Can you work these out from the drawing? Everything is in mm from the part's minimum corner. Coordinates: 2 decimals unless noted, no trailing zeros. Order: outer loops, then holes, each group sorted by start corner. A loop starts at its lowest first (then second) coordinate and runs counter-clockwise, first axis right, second up. Notation, with made-up numbers: M 28,71 L 67,71 A20 cw 67,95 Z; hole C 9.25,9.25 d11. An arc over 180 degrees is marked long. Answer as a JSON object with one key per item and string values.
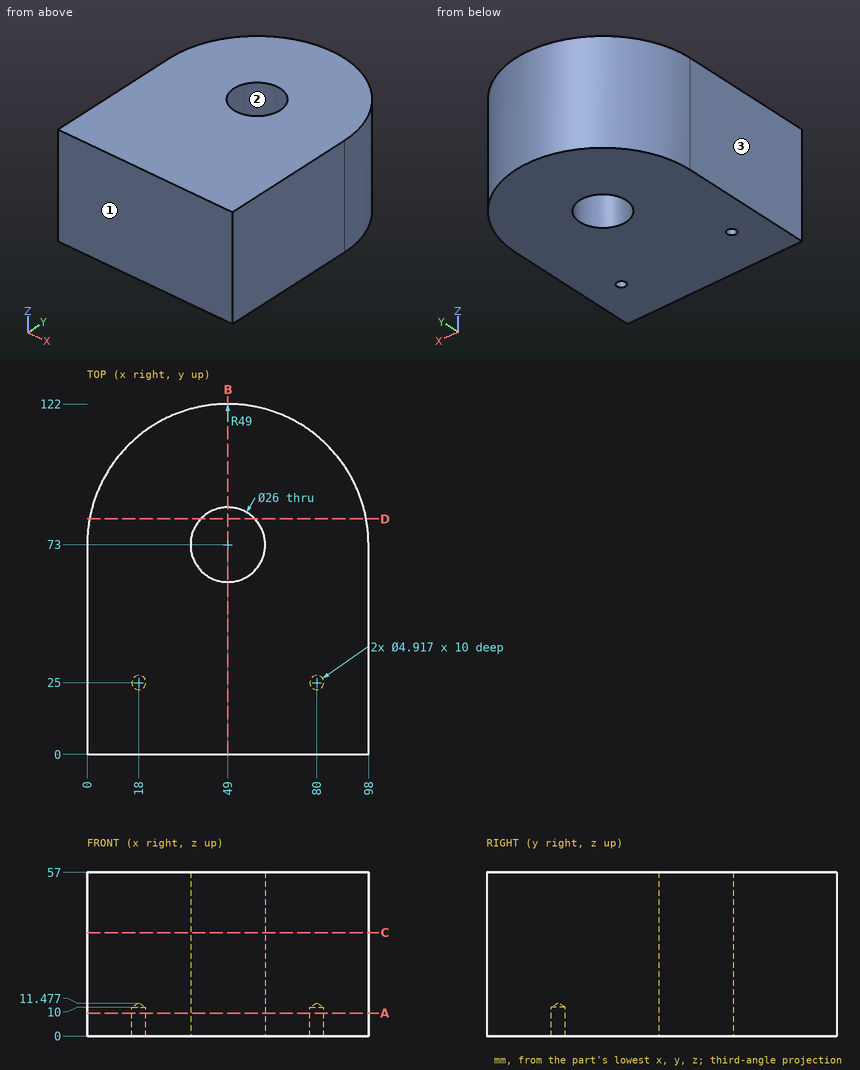
Item 1: I want a section at A-A, the plane z = 8. Write out the boundary of the cut face in (x, y), plus the area to 3 significant figures.
Answers follow:
{"outline": "M 0,0 L 98,0 L 98,73 A49 ccw 0,73 Z; hole C 18,25 d4.92; hole C 49,73 d26; hole C 80,25 d4.92", "area": "10,400 mm^2"}
Item 2: I want a section at B-B, the plane x = 49. Write out the boundary of the cut face in (y, z), plus the area to 3 significant figures.
Answers follow:
{"outline": "M 0,0 L 60,0 L 60,57 L 0,57 Z; M 86,0 L 122,0 L 122,57 L 86,57 Z", "area": "5,470 mm^2"}
Item 3: Please list where these lines run through material, in increasing order: line 1 (X direction, y = 25, z = 5.75); line 2 (X direction, y = 24.5, z = 7); line 3 (Y direction, x = 49, z = 24.5).
Answers follow:
{"line 1": "x = 0 to 15.54, 20.46 to 77.54, 82.46 to 98", "line 2": "x = 0 to 15.59, 20.41 to 77.59, 82.41 to 98", "line 3": "y = 0 to 60, 86 to 122"}
Item 4: I want a section at D-D, the plane y = 82. Write out the boundary of the cut face in (x, z), plus the area to 3 significant figures.
Answers follow:
{"outline": "M 0.83,0 L 39.62,0 L 39.62,57 L 0.83,57 Z; M 58.38,0 L 97.17,0 L 97.17,57 L 58.38,57 Z", "area": "4,420 mm^2"}
Item 5: I want a section at C-C, the plane z = 36. Write out the boundary of the cut face in (x, y), plus the area to 3 significant figures.
Answers follow:
{"outline": "M 0,0 L 98,0 L 98,73 A49 ccw 0,73 Z; hole C 49,73 d26", "area": "10,400 mm^2"}
Item 6: If we mould it in two halves opening along Y, with no side actions, what happens to the marked faces 1, 2 and 3? For each: pulls with the +Y half, pulls with the -Y half, needs draft (parallel to the pull), parting line crosses it, or undercut.
Answers follow:
{"face 1": "pulls with the -Y half", "face 2": "undercut", "face 3": "needs draft"}
Item 7: I'm going to push flat-ended pins straight in: pin 1 (4 mm diameter, centred on x = 18, y = 25, fed in from -Z) (1 decimal); pin 2 (12 mm diameter, centred on x = 50.5, z = 37.5, fed in from +Y); pin 3 (5 mm diameter, centred on y = 95.5, z = 29, fed in from +X). Where does each tip first touch, or does it pass through?
Answers follow:
{"pin 1": "stops at z = 10.3", "pin 2": "stops at y = 122", "pin 3": "stops at x = 93.73"}
